```python
from build123d import *

# Parameters (mm, degrees)
F0_R          = 19.05
F1_DEPTH      = 31.75
F2_R          = 9.525
F4_DEPTH      = 4.7752
F4_DEPTH_BACK = 15.875
F5_R          = 5.5626
F6_DEPTH      = 25.4


with BuildPart() as f1:
    # F0 (on Front) → F1 (new body, symmetric)
    with BuildSketch(Plane.XZ):
        with BuildLine():
            ThreePointArc((-27.491588, 62.326304), (-47.697164, 13.545728), (1.083412, 33.751304))
            ThreePointArc((1.083412, 33.751304), (-7.286012, 53.95688), (-27.491588, 62.326304))
        make_face()
        with Locations((-27.491588, 33.751304)):
            Circle(F0_R, mode=Mode.SUBTRACT)
        with BuildLine():
            ThreePointArc((-27.491588, 62.326304), (-7.286012, 53.95688), (1.083412, 33.751304))
            Line((1.083412, 33.751304), (1.083412, 46.451304))
            Line((1.083412, 46.451304), (42.358412, 46.451304))
            Line((42.358412, 46.451304), (42.358412, 62.326304))
            Line((42.358412, 62.326304), (-27.491588, 62.326304))
        make_face()
    extrude(amount=F1_DEPTH, both=True)

    # F2
    f2_edges = [f1.edges().sort_by_distance(p)[0] for p in [
        (1.083412, 0, 46.451304),
    ]]
    fillet(f2_edges, radius=F2_R)

    # F3 (on face) → F4 (join, two sides)
    with BuildSketch(Plane.XY.offset(62.326304)) as f4_sk:
        with BuildLine():
            ThreePointArc((27.853196, 30.077721), (15.178669, 30.033835), (8.854041, 19.05))
            Line((8.854041, 19.05), (8.854041, -19.05))
            ThreePointArc((8.854041, -19.05), (15.178669, -30.033835), (27.853196, -30.077721))
            Line((27.853196, -30.077721), (61.203396, -11.027721))
            ThreePointArc((61.203396, -11.027721), (67.604241, 0), (61.203396, 11.027721))
            Line((61.203396, 11.027721), (27.853196, 30.077721))
        make_face()
    extrude(amount=F4_DEPTH)
    extrude(f4_sk.sketch, amount=-F4_DEPTH_BACK)

    # F5 (on face) → F6 (cut)
    with BuildSketch(Plane.XY.offset(67.101504)):
        with Locations((21.554041, 19.05)):
            Circle(F5_R)
        with Locations((21.554041, -19.05)):
            Circle(F5_R)
        with Locations((54.904241, 0)):
            Circle(F5_R)
    extrude(amount=-F6_DEPTH, mode=Mode.SUBTRACT)


solid = f1.part
```
Input: part model. Units: mm. Frame: model coordinates. A direction names the side the tool comes from. Give positions to 0.01 mm unless a question says otherwise; leave off trailing zeros. Order: outer loops, then holes, each group sorted by start corner. A loop starts at its lowest first (then second) coordinate and runs counter-clockwise, first axis right, second up.
1. Section D-D on x = -18.5. Return the cut outline in (y, z).
Derived:
outline: (-31.75, 6.63) - (31.75, 6.63) - (31.75, 16.96) - (-31.75, 16.96) - close; (-31.75, 50.55) - (31.75, 50.55) - (31.75, 62.33) - (-31.75, 62.33) - close
2. Mould query, pull axis Y, two halves, no side actions, for faces 6 (the flat face through (37, -28, 62.326)), 7 (the cylindrical face through (15.34, 30.126, 64.68)), 8 (the flat face through (-8, -31.75, 41)), 9 (the cylindrical face through (15.997, -18.805, 56.921)). Classes: released by +Y, released by -Y, zero draft, split by the parting line, or undercut.
Derived:
face 6: zero draft
face 7: released by +Y
face 8: released by -Y
face 9: undercut
3. Section C-C on z = 50. Return the cut outline in (x, y).
Derived:
outline: (-51, -31.75) - (-37.44, -31.75) - (-37.44, 31.75) - (-51, 31.75) - close; (-17.55, -31.75) - (42.36, -31.75) - (42.36, -21.79) - (61.2, -11.03) arc R12.7 ccw to (61.2, 11.03) - (42.36, 21.79) - (42.36, 31.75) - (-17.55, 31.75) - close; hole circle Ø11.13 at (21.55, -19.05); hole circle Ø11.13 at (21.55, 19.05); hole circle Ø11.13 at (54.9, 0)
4. Section B-B on z = 29. Return the cut outline in (x, y).
Derived:
outline: (-55.67, -31.75) - (-45.94, -31.75) - (-45.94, 31.75) - (-55.67, 31.75) - close; (-9.04, -31.75) - (0.69, -31.75) - (0.69, 31.75) - (-9.04, 31.75) - close
5. Section A-A on y = 3.5. Give the number of separate pieces and of enclosed holes in the cut face, and give its area (3 significant figures).
Derived:
separate pieces: 2
enclosed holes: 1
area: 2,770 mm2
6. Pin query (flat end, axial travel): pin 1 (5 mm diameter, centred on x = 35.5, y = -26.5, fed in from +Z); pin 2 (1.4 mm diameter, centred on y = 8.5, z = 64.5, fed in from -X); pin 3 (6 mm diameter, centred on y = -0.5, z = 29, fed in from -X); pin 4 (3 mm diameter, centred on y = 25.5, z = 52.5, fed in from +X). Return the tip coordinate at first contact, or that it passes through.
Derived:
pin 1: stops at z = 67.1
pin 2: stops at x = 8.85
pin 3: stops at x = -56.01
pin 4: stops at x = 42.36
7. Material intervals for L1, parallel to Z at x = -28.5, y = 21; L2, parallel to Y at x = 25, z = 55; L3, parallel to Z at x = 51, y = -8, sorted ascending.
Derived:
L1: z = 5.19 to 14.73, 52.77 to 62.31
L2: y = -31.75 to -23.42, -14.68 to 14.68, 23.42 to 31.75
L3: z = 46.45 to 67.1
8. Reachability of faces 1 (the flat face through (8.854, 0, 65)), 2 (the flat face through (-8, 31.75, 41)), 3 (the flat face through (42.358, 27, 54)), 4 (the flat face through (37, 29, 62.326)), 5 (the flat face through (1.083, 0, 35)) from +Z, -Z, +X, -X, +Y, -Y: full face, straight path, thin tool, end or side. Return the list, or none.
Derived:
face 1: +Z, -X, +Y, -Y
face 2: +Z, -Z, +X, -X, +Y
face 3: +Z, -Z, +X, +Y
face 4: +Z, +X, +Y
face 5: -Z, +X, +Y, -Y
